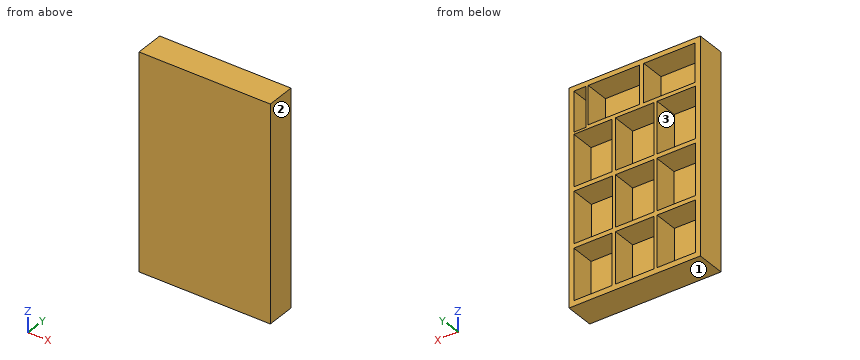
Autodesk Inventor part; units mm, degrees
ref_plane "YZ Plane" through (0, 0, 0) normal (1, 0, 0) x (0, 1, 0)
ref_plane "XZ Plane" through (0, 0, 0) normal (0, 1, 0) x (-1, 0, 0)
ref_plane "XY Plane" through (0, 0, 0) normal (0, 0, 1) x (1, 0, 0)
sketch "Эскиз1" plane through (0, 0, 0) normal (0, 1, 0) x (-1, 0, 0)
  line L0 (-41, -75) -> (41, -75)
  line L1 (41, -75) -> (41, 75)
  line L2 (41, 75) -> (-41, 75)
  line L3 (-41, 75) -> (-41, -75)
  line L4 (-41, -75) -> (41, 75) construction
  line L5 (41, -75) -> (-41, 75) construction
  line L6 (41, 75) -> (-41, 75)
  line L7 (-41, 75) -> (-41, 80)
  line L8 (-41, 80) -> (41, 80)
  line L9 (41, 80) -> (41, 75)
  point P0 (0, 0)
  point P1 (-45, 75)
  dimension "d0" = 150
  dimension "d1" = 82
  dimension "d34" = 5
extrude "Выдавливание1" add sketch "Эскиз1" along normal blind 3
sketch "Эскиз2" plane through (0, 3, 0) normal (0, 1, 0) x (1, 0, 0)
  line L0 (41, 75) -> (-41, 75)
  line L1 (43.9412, 73.2353) -> (-45, -75) construction
  line L2 (-45, 75) -> (45, -75) construction
  line L3 (38, 67.4874) -> (-38, 67.4874)
  line L4 (-38, 67.4874) -> (-38, -67.4874)
  line L5 (38, -67.4874) -> (38, 67.4874)
  line L6 (38, 67.4874) -> (-38, -67.4874) construction
  line L7 (-38, 67.4874) -> (38, -67.4874) construction
  line L8 (40.7632, -80) -> (-41, -80)
  line L9 (-38, -77) -> (-38, -67.4874)
  line L10 (41, -80) -> (41, 75)
  line L11 (41, -80) -> (-41, -80)
  line L12 (-41, 75) -> (-41, -80)
  line L13 (-41, -80) -> (41, -80)
  line L14 (38, -77) -> (-38, -77)
  line L15 (-41, -77) -> (-41, -80)
  line L16 (-41, -77) -> (-41, 75)
  line L17 (41, -80) -> (41, 75)
  line L18 (38, -67.4874) -> (38, -77)
  point P0 (0, 0)
  dimension "d38" = 3
  dimension "d39" = 3
extrude "Выдавливание2" add sketch "Эскиз2" along normal blind 15
sketch "Эскиз3" plane through (0, 3, 0) normal (0, 1, 0) x (1, 0, 0)
  line L0 (12, -16) -> (-12, -16)
  line L1 (-12, -16) -> (-12, 16)
  line L2 (-12, 16) -> (12, 16)
  line L3 (12, 16) -> (12, -16)
  line L4 (12, -16) -> (-12, 16) construction
  line L5 (-12, -16) -> (12, 16) construction
  line L6 (13, -17.3333) -> (-13, -17.3333)
  line L7 (-13, -17.3333) -> (-13, 17.3333)
  line L8 (-13, 17.3333) -> (13, 17.3333)
  line L9 (13, 17.3333) -> (13, -17.3333)
  line L10 (13, -17.3333) -> (-13, 17.3333) construction
  line L11 (-13, -17.3333) -> (13, 17.3333) construction
  point P0 (0, 0)
  dimension "d8" = 24
  dimension "d9" = 32
  dimension "d10" = 26
extrude "Выдавливание3" add sketch "Эскиз3" along normal blind 15
sketch "Эскиз4" plane through (0, 3, 0) normal (0, 1, 0) x (1, 0, 0)
  line L0 (13, 17.3333) -> (-13, 17.3333)
  line L1 (-13, 17.3333) -> (-39, 17.3333)
  line L2 (-39, 17.3333) -> (-39, -17.3333)
  line L3 (-39, -17.3333) -> (-13, -17.3333)
  line L4 (-13, -17.3333) -> (-13, 17.3333)
  line L5 (-13.8323, -16) -> (-37.8323, -16)
  line L6 (-37.8323, -16) -> (-37.8323, 16)
  line L7 (-37.8323, 16) -> (-13.8323, 16)
  line L8 (-13.8323, 16) -> (-13.8323, -16)
  line L9 (-13.8323, -16) -> (-37.8323, 16) construction
  line L10 (-37.8323, -16) -> (-13.8323, 16) construction
  line L11 (0, 0) -> (0, 60.0549)
  line L12 (13, 17.3333) -> (39, 17.3333)
  line L13 (39, 17.3333) -> (39, -17.3333)
  line L14 (39, -17.3333) -> (13, -17.3333)
  line L15 (13, -17.3333) -> (13, 17.3333)
  line L16 (13.8323, -16) -> (37.8323, -16)
  line L17 (37.8323, -16) -> (37.8323, 16)
  line L18 (37.8323, 16) -> (13.8323, 16)
  line L19 (13.8323, 16) -> (13.8323, -16)
  line L20 (13.8323, -16) -> (37.8323, 16) construction
  line L21 (37.8323, -16) -> (13.8323, 16) construction
  point P0 (-25.8323, 0)
  point P1 (25.8323, 0)
  dimension "d13" = 26
  dimension "d14" = 24
  dimension "d15" = 32
extrude "Выдавливание4" add sketch "Эскиз4" along normal blind 15
sketch "Эскиз6" plane through (0, 3, 0) normal (0, 1, 0) x (1, 0, 0)
  line L0 (38, 17.3333) -> (-38, 17.3333)
  line L1 (-39, 17.3333) -> (39, 17.3333)
  line L2 (39, 17.3333) -> (39, 52)
  line L3 (39, 52) -> (-39, 52)
  line L4 (-39, 52) -> (-39, 17.3333)
  line L5 (-39, 17.3333) -> (-13, 17.3333)
  line L6 (-13, 17.3333) -> (-13, 52)
  line L7 (-13, 52) -> (-39, 52)
  line L8 (-39, 52) -> (-39, 17.3333)
  line L9 (-14, 50.6667) -> (-38, 50.6667)
  line L10 (-38, 50.6667) -> (-38, 18.6667)
  line L11 (-38, 18.6667) -> (-14, 18.6667)
  line L12 (-14, 18.6667) -> (-14, 50.6667)
  line L13 (-14, 50.6667) -> (-38, 18.6667) construction
  line L14 (-38, 50.6667) -> (-14, 18.6667) construction
  line L15 (-39, 17.3333) -> (-13, 52)
  line L16 (-39, 52) -> (-13, 17.3333)
  line L17 (0, 0) -> (0, 94.2737)
  line L18 (39, 52) -> (39, 17.3333)
  line L19 (39, 17.3333) -> (13, 17.3333)
  line L20 (13, 17.3333) -> (13, 52)
  line L21 (13, 52) -> (39, 52)
  line L22 (39, 52) -> (39, 17.3333)
  line L23 (14, 50.6667) -> (38, 50.6667)
  line L24 (38, 50.6667) -> (38, 18.6667)
  line L25 (38, 18.6667) -> (14, 18.6667)
  line L26 (14, 18.6667) -> (14, 50.6667)
  line L27 (14, 50.6667) -> (38, 18.6667) construction
  line L28 (38, 50.6667) -> (14, 18.6667) construction
  line L29 (39, 17.3333) -> (13, 52)
  line L30 (39, 52) -> (13, 17.3333)
  line L31 (-13, 17.3333) -> (13, 17.3333)
  line L32 (13, 17.3333) -> (13, 52)
  line L33 (13, 52) -> (-13, 52)
  line L34 (-13, 52) -> (-13, 17.3333)
  line L35 (12, 50.6667) -> (-12, 50.6667)
  line L36 (-12, 50.6667) -> (-12, 18.6667)
  line L37 (-12, 18.6667) -> (12, 18.6667)
  line L38 (12, 18.6667) -> (12, 50.6667)
  line L39 (12, 50.6667) -> (-12, 18.6667) construction
  line L40 (-12, 50.6667) -> (12, 18.6667) construction
  line L41 (0, 0) -> (-32.6399, 0)
  line L42 (39, -17.3333) -> (-39, -17.3333)
  line L43 (-39, -17.3333) -> (39, -17.3333)
  line L44 (39, -17.3333) -> (39, -52)
  line L45 (39, -52) -> (-39, -52)
  line L46 (-39, -52) -> (-39, -17.3333)
  line L47 (-39, -17.3333) -> (-13, -17.3333)
  line L48 (-13, -17.3333) -> (-13, -52)
  line L49 (-13, -52) -> (-39, -52)
  line L50 (-39, -52) -> (-39, -17.3333)
  line L51 (-14, -50.6667) -> (-38, -50.6667)
  line L52 (-38, -50.6667) -> (-38, -18.6667)
  line L53 (-38, -18.6667) -> (-14, -18.6667)
  line L54 (-14, -18.6667) -> (-14, -50.6667)
  line L55 (-14, -50.6667) -> (-38, -18.6667) construction
  line L56 (-38, -50.6667) -> (-14, -18.6667) construction
  line L57 (-39, -17.3333) -> (-13, -52)
  line L58 (-39, -52) -> (-13, -17.3333)
  line L59 (39, -17.3333) -> (13, -17.3333)
  line L60 (38, -18.6667) -> (14, -18.6667)
  line L61 (14, -50.6667) -> (38, -50.6667)
  line L62 (38, -50.6667) -> (38, -18.6667)
  line L63 (14, -18.6667) -> (14, -50.6667)
  line L64 (14, -50.6667) -> (38, -18.6667) construction
  line L65 (38, -50.6667) -> (14, -18.6667) construction
  line L66 (39, -17.3333) -> (13, -52)
  line L67 (39, -52) -> (39, -17.3333)
  line L68 (13, -52) -> (39, -52)
  line L69 (39, -52) -> (39, -17.3333)
  line L70 (39, -52) -> (13, -17.3333)
  line L71 (13, -17.3333) -> (13, -52)
  line L72 (-13, -17.3333) -> (13, -17.3333)
  line L73 (13, -17.3333) -> (13, -52)
  line L74 (13, -52) -> (-13, -52)
  line L75 (-13, -52) -> (-13, -17.3333)
  line L76 (12, -50.6667) -> (-12, -50.6667)
  line L77 (-12, -50.6667) -> (-12, -18.6667)
  line L78 (-12, -18.6667) -> (12, -18.6667)
  line L79 (12, -18.6667) -> (12, -50.6667)
  line L80 (12, -50.6667) -> (-12, -18.6667) construction
  line L81 (-12, -50.6667) -> (12, -18.6667) construction
  point P0 (-26, 34.6667)
  point P1 (26, 34.6667)
  point P2 (0, 34.6667)
  point P3 (-26, -34.6667)
  point P4 (26, -34.6667)
  point P5 (0, -34.6667)
  dimension "d18" = 34.6667
  dimension "d19" = 26
  dimension "d20" = 24
  dimension "d21" = 32
  dimension "d22" = 24
extrude "Выдавливание5" add sketch "Эскиз6" along normal blind 15 contours L0 L30 L25 L29 L1 | L0 L17 L37 L38 L35 L3 L20 | L20 L29 L26 L30 | L29 L24 L30 L2 | L0 L6 L3 L17 L35 L36 L37 | L3 L30 L23 L29 | L16 L12 L15 L6 | L0 L1 L15 L11 L16 | L15 L9 L16 L3 | L4 L16 L10 L15 | L66 L60 L70 L42 | L44 L70 L62 L66 | L71 L45 L48 L42 | L70 L63 L66 L71 | L45 L66 L61 L70 | L58 L53 L57 L42 | L48 L57 L54 L58 | L57 L52 L58 L46 | L45 L58 L51 L57
sketch "Эскиз7" plane through (0, 3, 0) normal (0, 1, 0) x (1, 0, 0)
  line L0 (-37.6667, -53) -> (-5.6667, -53)
  line L1 (-5.6667, -53) -> (-5.6667, -77)
  line L2 (-5.6667, -77) -> (-37.6667, -77)
  line L3 (-37.6667, -77) -> (-37.6667, -53)
  line L4 (-4.3333, -52) -> (-39, -52)
  line L5 (-39, -52) -> (-39, -78)
  line L6 (-39, -78) -> (-4.3333, -78)
  line L7 (-4.3333, -78) -> (-4.3333, -52)
  line L8 (-4.3333, -52) -> (-39, -78) construction
  line L9 (-39, -52) -> (-4.3333, -78) construction
  line L10 (-37.6667, -77) -> (-5.6667, -53)
  line L11 (-5.6667, -77) -> (-37.6667, -53)
  line L12 (-4.3333, -52) -> (30.3333, -52)
  line L13 (30.3333, -52) -> (30.3333, -78)
  line L14 (30.3333, -78) -> (-4.3333, -78)
  line L15 (-4.3333, -78) -> (-4.3333, -52)
  line L16 (29, -53) -> (-3, -53)
  line L17 (-3, -53) -> (-3, -77)
  line L18 (-3, -77) -> (29, -77)
  line L19 (29, -77) -> (29, -53)
  line L20 (29, -53) -> (-3, -77) construction
  line L21 (-3, -53) -> (29, -77) construction
  line L22 (-4.3333, -78) -> (30.3333, -52)
  line L23 (30.3333, -78) -> (-4.3333, -52)
  point P0 (0, 0)
  point P1 (-21.6667, -65)
  point P2 (13, -65)
  dimension "d25" = 24
  dimension "d26" = 32
  dimension "d27" = 26
  dimension "d29" = 34.6667
  dimension "d30" = 34.6667
  dimension "d31" = 32
extrude "Выдавливание6" add sketch "Эскиз7" along normal blind 15 contours L7 L6 L5 L4 | L23 L17 L22 L7 | L12 L22 L16 L23 | L22 L18 L23 L14 | L13 L23 L19 L22
sketch "Эскиз8" plane through (0, 18, 0) normal (0, 1, 0) x (1, 0, 0)
  line L0 (-41, 75) -> (-41, -80)
  line L1 (-41, 75) -> (41.8498, 75)
  line L2 (41.8498, 75) -> (41.8498, 52)
  line L3 (41.8498, 52) -> (-41, 52)
  line L4 (-41, 52) -> (-41, 75)
  point P0 (0, 0)
  dimension "d40" = 23
extrude "Выдавливание7" cut sketch "Эскиз8" against normal blind 500
sketch "Эскиз9" plane through (0, 18, 0) normal (0, 1, 0) x (1, 0, 0)
  line L0 (-41, 52) -> (-41, -80)
  line L1 (-41, 52) -> (41, 52)
  line L2 (41, 52) -> (41, 54)
  line L3 (41, 54) -> (-41, 54)
  line L4 (-41, 54) -> (-41, 52)
  point P0 (0, 0)
  dimension "d43" = 2
extrude "Выдавливание8" add sketch "Эскиз9" against normal up to surface (18 mm away)
properties part number "хранитель крпелений"
Input: part model. Units: mm. Frame: model coordinates. Face numbers are marked on the shaded views. Coordinates: 2 decimals unless noted, no trailing zeros. Loops run counter-clockwise (first coordinate to the right, second up) from the corner with the lowest first, then second, coordinate; pieces in that order, holes last. Notation, with made-up numbers: M -1,-1.5 L 23,-1.5 A18 cw 23,17.5 Z; hole C 13.25,36 d10. An arc over 180 degrees is marked long. One line per item, written item: value.
(1) Section B-B (x = 3). Output: boundary loops of the cut face in (y, z), and give its area (3 significant figures).
Filled in:
outline: M 0,-54 L 18,-54 L 18,-50.67 L 3,-50.67 L 3,-18.67 L 18,-18.67 L 18,-16 L 3,-16 L 3,16 L 18,16 L 18,18.67 L 3,18.67 L 3,50.67 L 18,50.67 L 18,53 L 3,53 L 3,77 L 18,77 L 18,80 L 0,80 Z
area: 612 mm^2
(2) Section C-C (y = 5.25). Give the number of separate pieces and of enclosed holes in the cut face, and give its area (3 significant figures).
Filled in:
separate pieces: 1
enclosed holes: 12
area: 2,350 mm^2
(3) Section A-A (z = 61.5). Output: boundary loops of the cut face in (x, y).
Filled in:
outline: M -41,0 L 41,0 L 41,18 L 38,18 L 38,3 L 30.33,3 L 30.33,18 L 29,18 L 29,3 L -3,3 L -3,18 L -5.67,18 L -5.67,3 L -37.67,3 L -37.67,18 L -41,18 Z
(4) Section D-D (z = -1.5). Output: boundary loops of the cut face in (x, y).
Filled in:
outline: M -41,0 L 41,0 L 41,18 L 37.83,18 L 37.83,3 L 13.83,3 L 13.83,18 L 12,18 L 12,3 L -12,3 L -12,18 L -13.83,18 L -13.83,3 L -37.83,3 L -37.83,18 L -41,18 Z
(5) Pin query (flat end, axial travel): pin 1 (12 mm diameter, centred on x = -0.5, z = 38, fed in from +Y). Return the tip coordinate at first contact, or that it passes through.
Filled in:
pin 1: y = 3
(6) Pull-direction query (Z, two-part tool) for the marked faces 1, 2 and 3; classes: +Z half, -Z half, draft (parallel to the pull), parting line (faces both ways), or undercut.
Filled in:
face 1: -Z half
face 2: draft
face 3: undercut
(7) Line query: line 1 along X through (y, z) = (15.75, -43.5); line 2 along Z through (x, y) = (24, 11.25); line 3 along X through (y, z) = (12.5, 67). Output: solid intervals per line, ascending. Write a range as from..to.
Filled in:
line 1: -41..-38, -14..-12, 12..14, 38..41
line 2: -54..-50.67, -18.67..-16, 16..18.67, 50.67..53, 77..80
line 3: -41..-37.67, -5.67..-3, 29..30.33, 38..41
